Geometry check sheet. Reference: the model listing, model coordinates, mm. Face numbers are marked on the shaded views. A direction names the side the tool comes from. Give positions to 0.01 mm unless a question says otherwise; leave off trailing zeros. Order: outer loops, then holes, each group sorted by start corner. A loop starts at its lowest first (then second) coordinate and runs counter-clockwise, first axis right, second up. Notation, with made-up numbers: M 76,46.5 L 84,46.5 A7 cw 84,57.5 Z; hole C -13,-39 d10. An arc over 180 degrees is marked long. Answer as CSV lines item,"result". Start each with the question number.
Q1. Go/stop test with flat-tipped pins: pin 1 (5 mm diameter, centred on y = -28.5, z = -25.5, fed in from +X); pin 2 (15 mm diameter, centred on x = -10, y = -63, fed in from +Z). Record where each tip stops, or that it passes through.
Q2. Set-up check for the marked faces 1, 2 and 3: record each of +Z, -Z, +X, -X, +Y, -Y from which the full face is reachable in a straight line by a thin tool's end or side.
Q3. Thickness scan on line 1 (Z direction, x = 29, y = -79); line 2 (Z direction, x = -58, y = -56.5). Record the ranges inside material, lowest first.
Q4. Section check C-C, the plane z = -54. Record the boundary of the cut face in (x, y).
Q5. Section check D-D, the plane y = -15. Record the boundary of the cut face in (x, z).
Q6. Section check A-A, the plane x = 4. Record the boundary of the cut face in (y, z).
Q7. Section check B-B, the plane y = -51.5. Record the boundary of the cut face in (x, z), then the cut area to 3 significant figures.
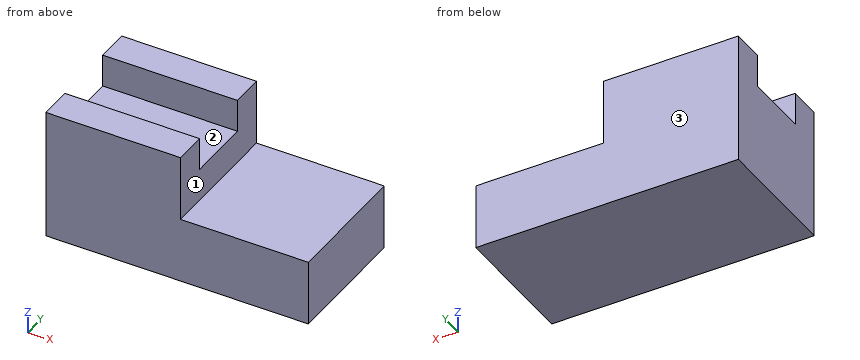
```python
from build123d import *

# Parameters (mm, degrees)
F1_DEPTH  = 101.6
F2_W      = 50.8
F2_H      = 25.4
F3_DEPTH  = 126.062407
F3_FACE_W = 50.8
F3_FACE_H = 25.4
F4_DEPTH  = 77.139593


with BuildPart() as f1:
    # F0 (on Front) → F1 (new body)
    with BuildSketch(Plane.XZ):
        Polygon((27.194744, -8.023955), (-77.138593, -8.023955), (-77.138593, -109.623955), (126.061407, -109.623955), (126.061407, -58.823955), (27.194744, -58.823955), align=None)
    extrude(amount=F1_DEPTH)

    # F2 (on Right) → F3 (cut, through all)
    with BuildSketch(Plane.YZ):
        with Locations((-50.8, -20.723955)):
            Rectangle(F2_W, F2_H)
    extrude(amount=F3_DEPTH, mode=Mode.SUBTRACT)

    # F3_face (on face) → F4 (cut, through all)
    with BuildSketch(Plane(origin=(0, -50.8, -20.723955), x_dir=(0, 1, 0), z_dir=(1, 0, 0))):
        Rectangle(F3_FACE_W, F3_FACE_H)
    extrude(amount=-F4_DEPTH, mode=Mode.SUBTRACT)


solid = f1.part
```
Answer block:
1,pin 1,"passes through"
1,pin 2,"stops at z = -33.42"
2,face 1,"+Z, +X, +Y, -Y"
2,face 2,"+Z, +X, -X"
2,face 3,"+Z, -Z, +X, -X, +Y"
3,line 1,"z = -109.62 to -58.82"
3,line 2,"z = -109.62 to -33.42"
4,outline,"M -77.14,-101.6 L 27.19,-101.6 L 27.19,0 L -77.14,0 Z"
5,outline,"M -77.14,-109.62 L 126.06,-109.62 L 126.06,-58.82 L 27.19,-58.82 L 27.19,-8.02 L -77.14,-8.02 Z"
6,outline,"M -101.6,-109.62 L 0,-109.62 L 0,-8.02 L -25.4,-8.02 L -25.4,-33.42 L -76.2,-33.42 L -76.2,-8.02 L -101.6,-8.02 Z"
7,outline,"M -77.14,-109.62 L 126.06,-109.62 L 126.06,-58.82 L 27.19,-58.82 L 27.19,-33.42 L -77.14,-33.42 Z"
7,area,"13,000 mm2"
